Input: part model. Units: mm. Frame: model coordinates. Round coordinates to 2 decimals unless told otherwise and drop trailing zeros. Write each loop counter-clockwise with the first axis right and the second up, starting at its lowest first coordinate (ties: lowest second). Pieces come first, ordered by that corner, then holes. Notation, with made-up numbers: (21.5, 23.5) -> (78.5, 23.5) arc R10 ccw to (78.5, 41.5) -> close; hole circle Ø3 at (-18, 0.25). An arc over 180 degrees is marked (long way). Write item = value, one per line. Start each with the question number.
```python
from build123d import *

# Parameters (mm, degrees)
SKETCH_R  = 2.1
PAD_DEPTH = 1


with BuildPart() as part:
    # Sketch → Pad (new body)
    with BuildSketch(Plane.XY):
        with BuildLine():
            Line((-5, 15), (3.5, 15))
            ThreePointArc((5, 13.5), (4.56066, 14.56066), (3.5, 15))
            Line((5, 13.5), (5, -3.5))
            ThreePointArc((3.5, -5), (4.56066, -4.56066), (5, -3.5))
            Line((3.5, -5), (-13.5, -5))
            ThreePointArc((-15, -3.5), (-14.56066, -4.56066), (-13.5, -5))
            Line((-15, -3.5), (-15, 5))
            ThreePointArc((-14.56066, 6.06066), (-14.885819, 5.574025), (-15, 5))
            Line((-14.56066, 6.06066), (-6.06066, 14.56066))
            ThreePointArc((-5, 15), (-5.574025, 14.885819), (-6.06066, 14.56066))
        make_face()
        with Locations((0, 10)):
            Circle(SKETCH_R, mode=Mode.SUBTRACT)
        with Locations((-10, 0)):
            Circle(SKETCH_R, mode=Mode.SUBTRACT)
        Circle(SKETCH_R, mode=Mode.SUBTRACT)
    extrude(amount=PAD_DEPTH)


solid = part.part
```
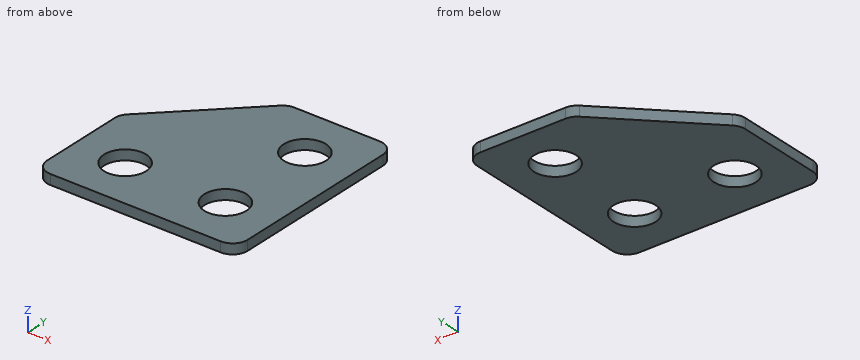
1. Section D-D (y = 10). Output: boundary loops of the cut face in (x, z).
2. Line query: line 1 along Y through (x, z) = (-0.5, 0.4); line 2 along Y through (x, z) = (-10, 0.5); line 3 along Y through (x, z) = (-8.75, 0.15). Output: solid intervals per line, ascending.
3. Pin query (flat end, axial travel): P1, Ø6.5, axis at x = -10, y = 0, coming from the -Z side. Return the tip coordinate at first contact, or that it passes through.
4. Section A-A (x = 0). Output: boundary loops of the cut face in (y, z), then the cut area to 3 significant figures.
5. Section C-C (z = 0.25). Output: boundary loops of the cut face in (x, y), then the cut area to 3 significant figures.
6. Section B-B (y = 0). Output: boundary loops of the cut face in (x, z).
Check sheet entries:
q1.outline = (-10.62, 0) -> (-2.1, 0) -> (-2.1, 1) -> (-10.62, 1) -> close; (2.1, 0) -> (5, 0) -> (5, 1) -> (2.1, 1) -> close
q2.line_1 = -5 to -2.04, 2.04 to 7.96, 12.04 to 15
q2.line_2 = -5 to -2.1, 2.1 to 10.62
q2.line_3 = -5 to -1.69, 1.69 to 11.87
q3.P1 = 0
q4.outline = (-5, 0) -> (-2.1, 0) -> (-2.1, 1) -> (-5, 1) -> close; (2.1, 0) -> (7.9, 0) -> (7.9, 1) -> (2.1, 1) -> close; (12.1, 0) -> (15, 0) -> (15, 1) -> (12.1, 1) -> close
q4.area = 11.6 mm2
q5.outline = (-15, -3.5) arc R1.5 ccw to (-13.5, -5) -> (3.5, -5) arc R1.5 ccw to (5, -3.5) -> (5, 13.5) arc R1.5 ccw to (3.5, 15) -> (-5, 15) arc R1.5 ccw to (-6.06, 14.56) -> (-14.56, 6.06) arc R1.5 ccw to (-15, 5) -> close; hole circle Ø4.2 at (-10, 0); hole circle Ø4.2 at (0, 0); hole circle Ø4.2 at (0, 10)
q5.area = 313 mm2
q6.outline = (-15, 0) -> (-12.1, 0) -> (-12.1, 1) -> (-15, 1) -> close; (-7.9, 0) -> (-2.1, 0) -> (-2.1, 1) -> (-7.9, 1) -> close; (2.1, 0) -> (5, 0) -> (5, 1) -> (2.1, 1) -> close
